Can you work these out from the model? Positions are in its coordinate system, mm. Face numbers are marked on the shaded views. Round coordinates to 2 decimals unless told otherwise and drop trailing zeros. Loops run counter-clockwise (first coordinate to the right, second up) from the corner with the lowest first, then second, coordinate; pieces in that order, holes last. Notation, with made-up numbers: M 11,19.5 L 35,19.5 A28 ccw 35,39.5 Z; hole C 68.25,21 d11. An arc over 180 degrees is marked long. Return JSON: item names as keys, results as strings.
Autodesk Inventor part; units mm, degrees
ref_plane "YZ Plane" through (0, 0, 0) normal (1, 0, 0) x (0, 1, 0)
ref_plane "XZ Plane" through (0, 0, 0) normal (0, 1, 0) x (-1, 0, 0)
ref_plane "XY Plane" through (0, 0, 0) normal (0, 0, 1) x (1, 0, 0)
sketch "Sketch1" plane through (0, 0, 0) normal (0, 1, 0) x (-1, 0, 0)
  line L0 (-2.4, 0) -> (2.4, 0)
  line L1 (2.4, 0) -> (2.4, 7.8)
  line L2 (2.4, 7.8) -> (-2.4, 7.8)
  line L3 (-2.4, 7.8) -> (-2.4, 0)
  arc A0 (-0.7, 4.9198) -> (0.7, 4.9198) centre (0, 3.65) ccw
  arc A1 (0.7, 4.9198) -> (-0.7, 4.9198) centre (0, 4.9959) ccw
  point P0 (0, 0)
  point P1 (0, 7.8)
  point P2 (0, 0)
  dimension "d0" = 4.8
  dimension "d1" = 7.8
  dimension "d2" = 5.6
  dimension "d3" = 1.45
  dimension "d4" = 2.1
  dimension "d5" = 1.4
extrude "Extrusion1" add sketch "Sketch1" along normal mid plane 0.85
chamfer "Chamfer1" distance 1.1 distance2 1 1 edges at (2.4, 0, 7.8) measured on face at (-0.8, -0.1417, 7.8)
chamfer "Chamfer2" distance 1.1 distance2 1 1 edges at (-2.4, 0, 7.8) measured on face at (0.0667, 0.1417, 7.8)
chamfer "Chamfer3" distance 1 distance2 0.175 1 edges at (0, 0.425, 7.8) measured on face at (0, 0.425, 0.7333)
chamfer "Chamfer4" distance 1 distance2 0.175 1 edges at (0, -0.425, 7.8) measured on face at (0, -0.425, 0.7333)
properties material "Nickel-Copper Alloy 400"
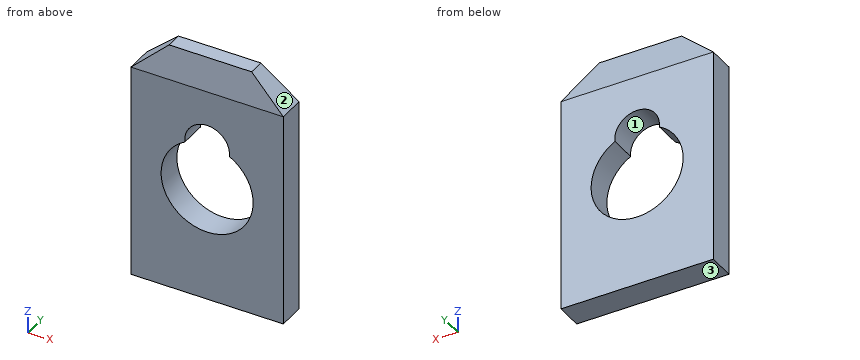
Q1. Suppose I cut it at C-C, the plane z = 4.75. Please give me the cut outline in (x, y) (3 decimals), plus the area to 3 significant figures.
Results:
{"outline": "M -2.4,-0.425 L -0.945,-0.425 L -0.945,0.425 L -2.4,0.425 Z; M 0.945,-0.425 L 2.4,-0.425 L 2.4,0.425 L 0.945,0.425 Z", "area": "2.47 mm2"}
Q2. I'm going to push a flat-ended pin straight in: pin 1 Ø0.8 at (x, z) = (0, 5) entering from +Y. Where does the tip first touch, or does it pass through?
Results:
{"pin 1": "passes through"}
Q3. Suppose I cut it at A-A, the plane y = -0.05. Please give me the cut outline in (x, z), plus the area to 3 significant figures.
Results:
{"outline": "M -2.4,0 L 2.4,0 L 2.4,6.8 L 1.3,7.8 L -1.3,7.8 L -2.4,6.8 Z; hole M -0.7,4.92 A1.45 ccw long 0.7,4.92 A0.7 ccw long Z", "area": "29.0 mm2"}
Q4. Suppose I cut it at B-B, the plane x = 0. Please give me the cut outline in (y, z) (3 decimals), plus the area to 3 significant figures.
Results:
{"outline": "M -0.425,0 L 0.425,0 L 0.425,2.2 L -0.425,2.2 Z; M -0.425,5.7 L 0.425,5.7 L 0.425,6.8 L 0.25,7.8 L -0.25,7.8 L -0.425,6.8 Z", "area": "3.48 mm2"}
Q5. Thinking about a two-plate mould opening in Z: for the marked faces 1, 2 and 3, which applies, pulls with the +Z half, pulls with the -Z half, needs draft (parallel to the pull), parting line crosses it, or undercut?
Results:
{"face 1": "undercut", "face 2": "pulls with the +Z half", "face 3": "pulls with the -Z half"}
Q6. If I drill on line 1 along Z through (x, y) = (0, 0); line 2 along X through (y, z) = (0.25, 5); line 3 along X through (y, z) = (0.1, 3.65), over which ranges is the centre line in solid material (lowest first)?
Results:
{"line 1": "z = 0 to 2.2, 5.7 to 7.8", "line 2": "x = -2.4 to -0.7, 0.7 to 2.4", "line 3": "x = -2.4 to -1.45, 1.45 to 2.4"}
Q7. Suppose I cut it at D-D, the plane x = 1. Please give me the cut outline in (y, z) (3 decimals).
Results:
{"outline": "M -0.425,0 L 0.425,0 L 0.425,2.6 L -0.425,2.6 Z; M -0.425,4.7 L 0.425,4.7 L 0.425,6.8 L 0.25,7.8 L -0.25,7.8 L -0.425,6.8 Z"}
